Input: part model. Units: mm. Frame: model coordinates. Coordinates: 2 decimals unless noted, no trailing zeros. Loops run counter-clockwise (first coordinate to the right, second up) from the corner with the lowest first, then second, coordinate; pieces in that order, holes last.
Item 1: Section A-A on y = 9. Return loops of the section in (x, z), and give its area (3 significant figures).
Item 2: Contact query for flat-ended pins moving along their axis: P1, Ø6, axis at y = 1, z = 2, coming from the -X side; P2, Ø12, axis at x = -17.5, y = -4, coming from the +Z side. Output: stop coordinate, or through.
Item 3: Section B-B on z = 4.75. Return loops of the section in (x, y), and give its area (3 significant figures).
Item 4: Ray query, line 1 along X through (y, z) = (-8.75, -2). Return the intervals inside material, ascending.
```python
from build123d import *

# Parameters (mm, degrees)
F1_DEPTH = 5.969
F2_DEPTH = 0.254


with BuildPart() as f1:
    # F0 (on Top) → F1 (new body, symmetric)
    with BuildSketch(Plane.XY):
        Polygon((11.1125, 11.1125), (-11.1125, 11.1125), (-11.1125, 0.254), (-11.1125, -0.254), (-11.1125, -11.1125), (11.1125, -11.1125), align=None)
    extrude(amount=F1_DEPTH, both=True)

    # F0 (on Top) → F2 (join, symmetric)
    with BuildSketch(Plane.XY):
        Polygon((-11.1125, -0.254), (-11.1125, 0.254), (-28.986987, 0.254), (-28.986987, 0), (-28.986987, -0.254), align=None)
    extrude(amount=F2_DEPTH, both=True)


solid = f1.part
```
Results found:
1. outline: (-11.11, -5.97) - (11.11, -5.97) - (11.11, 5.97) - (-11.11, 5.97) - close
1. area: 265 mm2
2. P1: stops at x = -28.99
2. P2: stops at z = 0.25
3. outline: (-11.11, -11.11) - (11.11, -11.11) - (11.11, 11.11) - (-11.11, 11.11) - close
3. area: 494 mm2
4. line 1: x = -11.11 to 11.11
